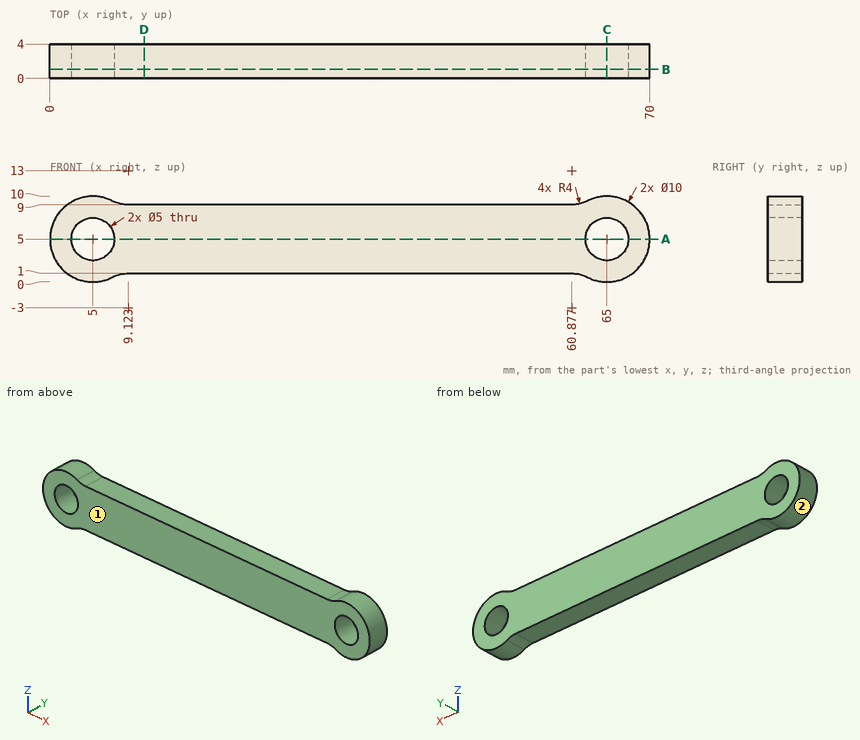
Input: dimensioned drawing with shaded views. Units: mm. Origin: part minimum x, y, z. Round coordinates to 2 decimals unless told otherwise and drop trailing zeros. Order: outer loops, then holes, each group sorted by start corner. A loop starts at its lowest first (then second) coordinate and runs counter-clockwise, first axis right, second up. Notation, with made-up numbers: (60.5, -34.5) - (89.5, -34.5) arc R30 ccw to (89.5, -1.5) - close; hole circle Ø9 at (82, -36). An arc over 180 degrees is marked (long way). Answer as a JSON object with one key per item and string values. Group by question number.
(1) Cut plane B-B (y = 1.05). Return loops of the section in (x, z).
(2) Cut plane A-A (z = 5). Return loops of the section in (x, y), then the cut area to 3 significant figures.
(3) Material intervals for probe 1 along X at (y, z) = (2.15, 5); probe 2 along Z at (x, y) = (65, 1.7); probe 3 along Z at (x, y) = (28.5, 1.55), sorted ascending. Write a range as from..to.
(4) Pin query (flat end, axial travel): P1, Ø4.5, axis at x = 5, z = 5, coming from the +Y side; P2, Ø2, axis at x = 12, y = 2.5, coming from the -Z side; P3, Ø1, axis at x = 46.5, y = 0.5, coming from the +Z side; P4, Ø1.5, axis at y = 3, z = 2, coming from the -X side (3 decimals). Return the tip coordinate at first contact, or that it passes through.
(5) Draft query along X for the marked faces 1 and 2. Return one class per face: released by +X, released by -X, zero draft, split by the parting line, or undercut.
(6) Cut plane C-C (x = 65). Return loops of the section in (y, z).
(7) Cut plane D-D (x = 11). Return loops of the section in (y, z), then the cut area to 3 significant figures.
Here are the results:
{
 "1": {"outline": "(7.29, 0.56) arc R4 cw to (9.12, 1) - (60.88, 1) arc R4 cw to (62.71, 0.56) arc R5 ccw (long way) to (62.71, 9.44) arc R4 cw to (60.88, 9) - (9.12, 9) arc R4 cw to (7.29, 9.44) arc R5 ccw (long way) to start; hole circle Ø5 at (5, 5); hole circle Ø5 at (65, 5)"},
 "2": {"outline": "(0, 0) - (2.5, 0) - (2.5, 4) - (0, 4) - close; (7.5, 0) - (62.5, 0) - (62.5, 4) - (7.5, 4) - close; (67.5, 0) - (70, 0) - (70, 4) - (67.5, 4) - close", "area": "240 mm^2"},
 "3": {"probe 1": "x = 0..2.5, 7.5..62.5, 67.5..70", "probe 2": "z = 0..2.5, 7.5..10", "probe 3": "z = 1..9"},
 "4": {"P1": "passes through", "P2": "stops at z = 1", "P3": "stops at z = 9", "P4": "stops at x = 0.535"},
 "5": {"face 1": "zero draft", "face 2": "undercut"},
 "6": {"outline": "(0, 0) - (4, 0) - (4, 2.5) - (0, 2.5) - close; (0, 7.5) - (4, 7.5) - (4, 10) - (0, 10) - close"},
 "7": {"outline": "(0, 1) - (4, 1) - (4, 9) - (0, 9) - close", "area": "32.0 mm^2"}
}
